```python
from build123d import *

# Parameters (mm, degrees)
F0_R     = 3.37312
F1_DEPTH = 2.54
F2_DEPTH = 6.477


with BuildPart() as f1:
    # F0 (on Top) → F1 (new body)
    with BuildSketch(Plane.XY):
        Polygon((5.54355, -3.20057), (5.54355, 3.20057), (0, 6.40114), (-5.54355, 3.20057), (-5.54355, -3.20057), (0, -6.40114), align=None)
        Circle(F0_R, mode=Mode.SUBTRACT)
    extrude(amount=F1_DEPTH)

    # F0 (on Top) → F2 (join)
    with BuildSketch(Plane.XY):
        Polygon((6.477, -3.739498), (6.477, 3.739498), (0, 7.478995), (-6.477, 3.739498), (-6.477, -3.739498), (0, -7.478995), align=None)
        Polygon((0, 6.40114), (5.54355, 3.20057), (5.54355, -3.20057), (0, -6.40114), (-5.54355, -3.20057), (-5.54355, 3.20057), align=None, mode=Mode.SUBTRACT)
    extrude(amount=F2_DEPTH)


solid = f1.part
```
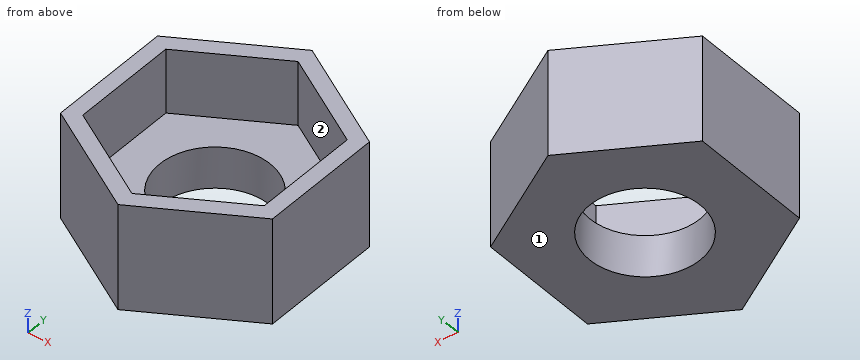
Here's how the part is built. I have some questions about the finished solid (model axes, mm). Face numbers are marked on the shaded views. A direction names the side the tool comes from. Give positions to 0.01 mm unless a question says otherwise; leave off trailing zeros. Order: outer loops, then holes, each group sorted by start corner. A loop starts at its lowest first (then second) coordinate and runs counter-clockwise, first axis right, second up. Notation, with made-up numbers: M 70,-2.75 L 107,-2.75 A20 ccw 107,30.25 Z; hole C 6,22 d11. An arc over 180 degrees is marked long. Use a Markdown table: item, result. Add a question column.
1. Suppose I cut it at A-A (y = 0). List the corners of the cut face in (x, z) for me, and give its area (3 significant figures).
2. I need wall thicknesses on probe 1 along X at (y, z) = (-0.5, 2.75); probe 2 along Z at (x, y) = (4, -3); probe 3 along X at (y, z) = (-5.5, 5.5). Which ranges of each line are inside material? Lowest first, please. Write a range as from..to.
3. Suppose I cut it at D-D (z = 2). List the corners of the cut face in (x, y) for me.
4. On a 3-axis mill with a long thin cutter (end or side, diameter ignored), from which of +Z, -Z, +X, -X, +Y, -Y can I reach the whole of each face in a straight line? I mean the marked faces 1 and 2. Say none if no direction works.
5. Suppose I cut it at C-C (x = 0.25). List the corners of the cut face in (y, z) for me, and give its area (3 significant figures).
6. Suppose I cut it at B-B (z = 4). List the corners of the cut face in (x, y) for me, and give its area (3 significant figures).
Results list:
| question | item | result |
|---|---|---|
| 1 | outline | M -6.48,0 L -3.37,0 L -3.37,2.54 L -5.54,2.54 L -5.54,6.48 L -6.48,6.48 Z; M 3.37,0 L 6.48,0 L 6.48,6.48 L 5.54,6.48 L 5.54,2.54 L 3.37,2.54 Z |
| 1 | area | 23.1 mm² |
| 2 | probe 1 | x = -6.48..-5.54, 5.54..6.48 |
| 2 | probe 2 | z = 0..2.54 |
| 2 | probe 3 | x = -3.43..-1.56, 1.56..3.43 |
| 3 | outline | M -6.48,-3.74 L 0,-7.48 L 6.48,-3.74 L 6.48,3.74 L 0,7.48 L -6.48,3.74 Z; hole C 0,0 d6.75 |
| 4 | face 1 | -Z, +X, -X, +Y, -Y |
| 4 | face 2 | +Z |
| 5 | outline | M -7.33,0 L -3.36,0 L -3.36,2.54 L -6.26,2.54 L -6.26,6.48 L -7.33,6.48 Z; M 3.36,0 L 7.33,0 L 7.33,6.48 L 6.26,6.48 L 6.26,2.54 L 3.36,2.54 Z |
| 5 | area | 28.7 mm² |
| 6 | outline | M -6.48,-3.74 L 0,-7.48 L 6.48,-3.74 L 6.48,3.74 L 0,7.48 L -6.48,3.74 Z; hole M -5.54,-3.2 L 0,-6.4 L 5.54,-3.2 L 5.54,3.2 L 0,6.4 L -5.54,3.2 Z |
| 6 | area | 38.9 mm² |
